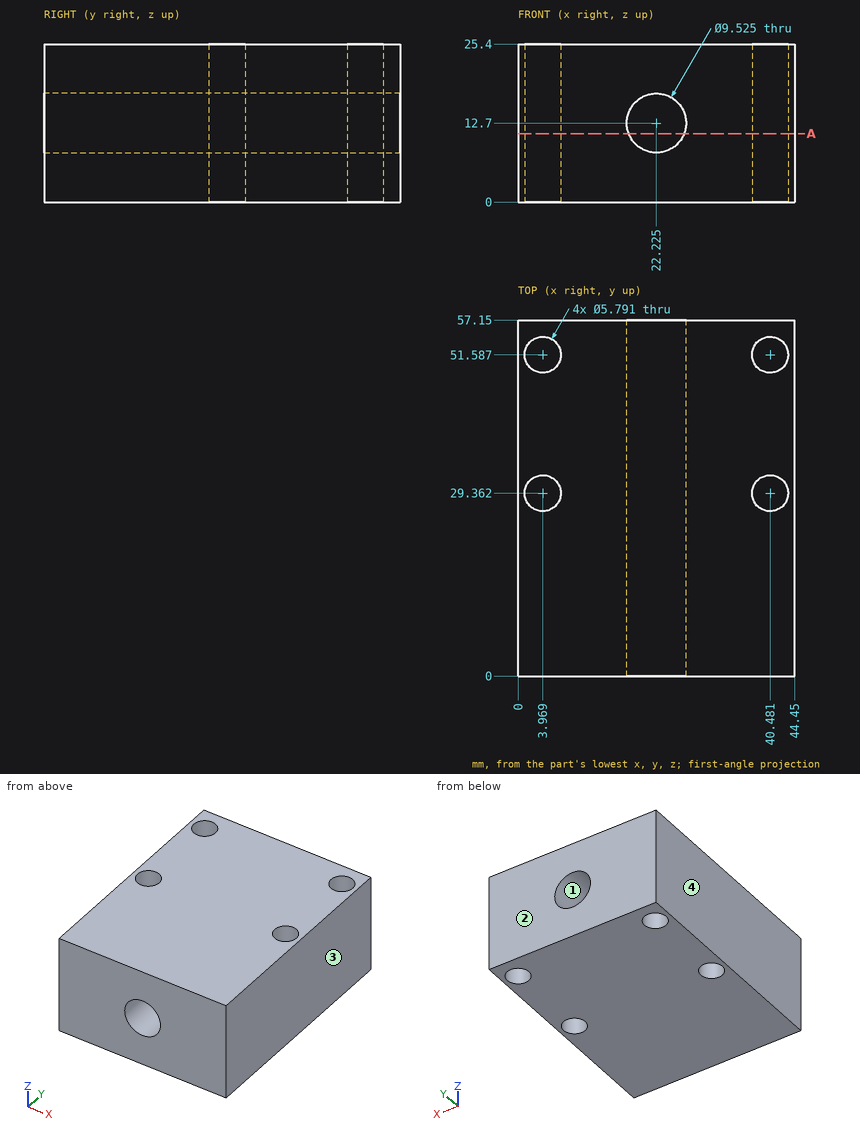
Check sheet for the drawn part. Datum: minimum x, y, z corner. Units: mm. Round coordinates to 2 decimals unless told otherwise and drop trailing zeros.
(1) Scan lines: probe 1 along X at (y, z) = (18.5, 13); probe 2 along Z at (x, y) = (21, 20); probe 3 along X at (y, z) = (17.5, 14.25). Record each from-to range of solid material in increasing order.
(2) Draft check along X on the marked faces 1, 2, 3 and 4. Enter one of: pulls with the +X half, pulls with the -X half, needs draft (parallel to the pull), parting line crosses it, or undercut.
(3) Cross-section at A-A, the plane z = 11. State how many separate pieces and enclosed holes the cut face has, and give its area (3 significant figures).
Check sheet entries:
1. probe 1: x = 0 to 17.47, 26.98 to 44.45
1. probe 2: z = 0 to 8.1, 17.3 to 25.4
1. probe 3: x = 0 to 17.72, 26.73 to 44.45
2. face 1: undercut
2. face 2: needs draft
2. face 3: pulls with the +X half
2. face 4: pulls with the -X half
3. separate pieces: 2
3. enclosed holes: 4
3. area: 1,930 mm2
